Build history of the part. All positions in model axes, mm. A direction names the side the tool comes from. Coordinates: 2 decimals unless noted, no trailing zeros. Write each loop counter-clockwise with the first axis right and the second up, starting at its lowest first coordinate (ties: lowest second). Pieces come first, ordered by that corner, then holes. Notation, with made-up numbers: (-28, -24) -> (-6, -24) arc R32 cw to (-6, 10) -> close; hole circle Ø4 at (-27.5, 31). An arc over 180 degrees is marked (long way). Write each question's results on one line, items separated by ' | '. Start each with the question number.
Q1. Saw through at B-B on x = 88. Give the cut face in (y, z).
Q2. Drop flat-ended pins along their axis: pin 1 Ø3 at (x, y) = (72.32, 145) entering from -Z; pin 2 Ø0.5 at (x, z) = (50, 0.5) entering from -Y; pin 3 Ø4.5 at (x, y) = (80.76, 75) entering from +Z; pin 4 Ø10 at (x, y) = (70.5, 54.5) entering from +Z. Give the stop position or say it passes through.
Q3. Two-plate mould, pull along Y, no slides. Class faces 1 (the face through (24.65, 2.46, 43.1)), 2 (the face through (21.011, 75.923, 1.479)), 3 (the face through (82.54, 75.92, 1.48)), 4 (the face through (38, 0, 35)): released by +Y, released by -Y, zero draft, split by the parting line, or undercut.
Q4. Tool access for faces 5 (the face through (51, 140, 9)), 6 (the face through (0, 2, 14)): list every direction of +Z, -Z, +X, -X, +Y, -Y with a clear straight run to the whole face (end or side of a thin tool).
Q5. Drill centre lines: line 1 (X direction, y = 145, z = 2); line 2 (X direction, y = 75, z = 1.2); line 3 (Z direction, x = 15.5, y = 39). Where is each one in solid material? Low to high.
Q6. Saw through at A-A on y = 145. Give the cut face in (x, z), and give its area (3 significant figures).
Q7. Saw through at C-C on z = 42. Give the cut face in (x, y).
Q8. Saw through at D-D on y = 75. Count the separate pieces of the cut face and the enclosed holes in it, and give its area (3 significant figures).
from build123d import *

# Parameters (mm, degrees)
EXTRUDE002_DEPTH = 5
FACE007_R        = 2
EXTRUDE001_DEPTH = 10
EXTRUDE_DEPTH    = 3


with BuildPart() as extrude002:
    # Sketch008 (on Face18 of Cut001) → Extrude002 (new body)
    with BuildSketch(Plane.XZ):
        Polygon((0, 0), (0, 28.867513), (50, 57.735027), (100, 28.867513), (100, 0), (83, 0), (83, 19.052559), (50, 38.105118), (17, 19.052559), (17, 0), align=None)
    extrude(amount=-EXTRUDE002_DEPTH)


with BuildPart() as extrude001:
    # Face007 → Extrude001 (new body)
    with BuildSketch(Plane(origin=(88, 15, 0), x_dir=(0, 1, 0), z_dir=(0, 0, 1))):
        Circle(FACE007_R)
        with Locations((0, 76)):
            Circle(FACE007_R)
        with Locations((60, 68.763311)):
            Circle(FACE007_R)
        with Locations((60, 7.236689)):
            Circle(FACE007_R)
        with Locations((130, 15.679492)):
            Circle(FACE007_R)
        with Locations((130, 40.949188)):
            Circle(FACE007_R)
        with Locations((130, 60.320508)):
            Circle(FACE007_R)
    extrude(amount=EXTRUDE001_DEPTH)


with BuildPart() as loft002:
    # Face006 → Loft002 section 0
    with BuildSketch(Plane(origin=(50, 125, 7.409328), x_dir=(1, 0, 0), z_dir=(0, 1, 0))):
        Polygon((-16.5, 7.409328), (-16.5, -2.116951), (0, -11.64323), (16.5, -2.116951), (16.5, 7.409328), align=None)
    # Face005 → Loft002 section 1
    with BuildSketch(Plane(origin=(50, 130, 0.224525), x_dir=(1, 0, 0), z_dir=(0, 1, 0))):
        Polygon((-0.5, 0.224525), (-0.5, -0.06415), (0, -0.352825), (0.5, -0.06415), (0.5, 0.224525), align=None)
    loft()


with BuildPart() as fusion001:
    # Face003 → Loft001 section 0
    with BuildSketch(Plane(origin=(50, 125, 7.409328), x_dir=(1, 0, 0), z_dir=(0, 1, 0))):
        Polygon((-16.5, 7.409328), (-16.5, -2.116951), (0, -11.64323), (16.5, -2.116951), (16.5, 7.409328), align=None)
    # Face004 → Loft001 section 1
    with BuildSketch(Plane(origin=(50, 0, 14.818657), x_dir=(1, 0, 0), z_dir=(0, 1, 0))):
        Polygon((-33, 14.818657), (-33, -4.233902), (0, -23.286461), (33, -4.233902), (33, 14.818657), align=None)
    loft()

    # Fusion001: union Loft002
    add(loft002.part)


with BuildPart() as loft_body:
    # Face001 → Loft section 0
    with BuildSketch(Plane(origin=(50, 0, 15.716757), x_dir=(1, 0, 0), z_dir=(0, 1, 0))):
        Polygon((35, 15.716757), (-35, 15.716757), (-35, -4.490502), (0, -24.697762), (35, -4.490502), align=None)
    # Face002 → Loft section 1
    with BuildSketch(Plane(origin=(50, 140, 7.777778), x_dir=(1, 0, 0), z_dir=(0, 1, 0))):
        Polygon((-17.320508, 7.777778), (-17.320508, -2.222222), (0, -12.222222), (17.320508, -2.222222), (17.320508, 7.777778), align=None)
    loft()


with BuildPart() as fusion002:
    # Face → Extrude (new body)
    with BuildSketch(Plane(origin=(50, 68.75, 0), x_dir=(0, 1, 0), z_dir=(0, 0, 1))):
        Polygon((-68.75, 50), (-68.75, -50), (81.25, -30), (81.25, 30), align=None)
    extrude(amount=EXTRUDE_DEPTH)

    # Fusion: union Loft body
    add(loft_body.part)

    # Cut: cut Fusion001
    add(fusion001.part, mode=Mode.SUBTRACT)

    # Cut001: cut Extrude001
    add(extrude001.part, mode=Mode.SUBTRACT)

    # Fusion002: union Extrude002
    add(extrude002.part)


solid = fusion002.part
Returned:
1) outline: (0, 0) -> (13, 0) -> (13, 3) -> (5, 3) -> (5, 35.8) -> (0, 35.8) -> close; (17, 0) -> (90, 0) -> (90, 3) -> (17, 3) -> close
2) pin 1: passes through | pin 2: stops at y = 129.94 | pin 3: stops at z = 3 | pin 4: stops at z = 23.61
3) face 1: zero draft | face 2: undercut | face 3: undercut | face 4: released by -Y
4) face 5: +Z, +X, -X, +Y | face 6: +Z, -Z, -X, +Y, -Y
5) line 1: x = 19.33 to 25.68, 29.68 to 45.05, 49.05 to 70.32, 74.32 to 80.67 | line 2: x = 10 to 17.24, 21.24 to 26.9, 73.1 to 78.76, 82.76 to 90 | line 3: z = 0 to 3
6) outline: (19.33, 0) -> (25.68, 0) -> (25.68, 3) -> (19.33, 3) -> close; (29.68, 0) -> (45.05, 0) -> (45.05, 3) -> (29.68, 3) -> close; (49.05, 0) -> (70.32, 0) -> (70.32, 3) -> (49.05, 3) -> close; (74.32, 0) -> (80.67, 0) -> (80.67, 3) -> (74.32, 3) -> close | area: 148 mm2
7) outline: (22.75, 0) -> (77.25, 0) -> (77.25, 5) -> (22.75, 5) -> close
8) separate pieces: 3 | enclosed holes: 0 | area: 267 mm2
